Autodesk Inventor part; units mm, degrees
ref_plane "YZ Plane" through (0, 0, 0) normal (1, 0, 0) x (0, 1, 0)
ref_plane "XZ Plane" through (0, 0, 0) normal (0, 1, 0) x (-1, 0, 0)
ref_plane "XY Plane" through (0, 0, 0) normal (0, 0, 1) x (1, 0, 0)
sketch "Sketch_1" plane through (0, 0, 0) normal (0, 0, 1) x (1, 0, 0)
  line L0 (6, 0) -> (-0.8, 0)
  line L1 (-0.8, 0) -> (-0.8, 2.7673)
  line L2 (-0.8, 2.7673) -> (-0.5333, 3.5)
  line L3 (-0.5333, 3.5) -> (0, 3.5)
  line L4 (0, 3.5) -> (0, 1.9)
  arc A0 (0, 1.9) -> (0.4, 1.5) centre (0.4, 1.9) ccw
  line L5 (0.4, 1.5) -> (6, 1.5)
  line L6 (6, 1.5) -> (6, 0)
  line L7 (6, 0) -> (-0.8, 0)
revolve "Revolution1" add sketch "Sketch_1" angle 360 about axis through (6, 0, 0) along (1, 0, 0)
thread "Thread1"
sketch "Sketch_5" plane through (-0.05, 0, 0) normal (1, 0, 0) x (0, 0, -1)
  arc A0 (-0.6801, -0.1159) -> (-0.4404, -0.531) centre (-0.5499, -0.3175) ccw
  arc A1 (-0.341, -0.5357) -> (-0.4404, -0.531) centre (-0.3947, -0.62) ccw
  arc A2 (-0.341, -0.5357) -> (-0.2934, -0.5632) centre (0, 0) ccw
  arc A3 (-0.2397, -0.6469) -> (-0.2934, -0.5632) centre (-0.3396, -0.6519) ccw
  arc A4 (-0.2397, -0.6469) -> (0.2397, -0.6469) centre (0, -0.635) ccw
  arc A5 (0.2934, -0.5632) -> (0.2397, -0.6469) centre (0.3396, -0.6519) ccw
  arc A6 (0.2934, -0.5632) -> (0.341, -0.5357) centre (0, 0) ccw
  arc A7 (0.4404, -0.531) -> (0.341, -0.5357) centre (0.3947, -0.62) ccw
  arc A8 (0.4404, -0.531) -> (0.6801, -0.1159) centre (0.5499, -0.3175) ccw
  arc A9 (0.6344, -0.0275) -> (0.6801, -0.1159) centre (0.7343, -0.0318) ccw
  arc A10 (0.6344, -0.0275) -> (0.6344, 0.0275) centre (0, 0) ccw
  arc A11 (0.6801, 0.1159) -> (0.6344, 0.0275) centre (0.7343, 0.0318) ccw
  arc A12 (0.6801, 0.1159) -> (0.4404, 0.531) centre (0.5499, 0.3175) ccw
  arc A13 (0.341, 0.5357) -> (0.4404, 0.531) centre (0.3947, 0.62) ccw
  arc A14 (0.341, 0.5357) -> (0.2934, 0.5632) centre (0, 0) ccw
  arc A15 (0.2397, 0.6469) -> (0.2934, 0.5632) centre (0.3396, 0.6519) ccw
  arc A16 (0.2397, 0.6469) -> (-0.2397, 0.6469) centre (0, 0.635) ccw
  arc A17 (-0.2934, 0.5632) -> (-0.2397, 0.6469) centre (-0.3396, 0.6519) ccw
  arc A18 (-0.2934, 0.5632) -> (-0.341, 0.5357) centre (0, 0) ccw
  arc A19 (-0.4404, 0.531) -> (-0.341, 0.5357) centre (-0.3947, 0.62) ccw
  arc A20 (-0.4404, 0.531) -> (-0.6801, 0.1159) centre (-0.5499, 0.3175) ccw
  arc A21 (-0.6344, 0.0275) -> (-0.6801, 0.1159) centre (-0.7343, 0.0318) ccw
  arc A22 (-0.6344, 0.0275) -> (-0.6344, -0.0275) centre (0, 0) ccw
  arc A23 (-0.6801, -0.1159) -> (-0.6344, -0.0275) centre (-0.7343, -0.0318) ccw
extrude "Extrusion1" cut sketch "Sketch_5" against normal blind 0.75
sketch "Sketch_2" plane through (0, 0, 0) normal (0, 0, 1) x (1, 0, 0)
  line L0 (0.4552, 0) -> (0, 0)
  line L1 (-0.05, 0) -> (-0.05, 0.875)
  line L2 (-0.05, 0.875) -> (0.4552, 0)
  line L3 (0.4552, 0) -> (-0.05, 0)
revolve "Revolution2" cut sketch "Sketch_2" angle 360 about axis through (0.4552, 0, 0) along (1, 0, 0)
properties part number "超極低頭ネジL6" material "ステンレス鋼"
Work out the finished part from the listing and answer in its coordinate system (mm). A direction names the side the tool comes from. Give positions to 0.01 mm unless a question says otherwise; leave off trailing zeros. Loops run counter-clockwise (first coordinate to the right, second up) from the corner with the lowest first, then second, coordinate; pieces in that order, holes last. Notation, with made-up numbers: (-32.75, 58) - (19.25, 58) arc R25 cw to (19.25, 74) - close; hole circle Ø1 at (32, -28.75). An arc over 180 degrees is marked (long way). Answer in a Markdown table with one row per item. Add a question column.
Q1. The part is cut by section A-A (x = 4). Determine the outline of the cut face in (y, z).
Q2. A tool of negligible diameter and unlimited length cuts with its end or side. For faces 1 (the flat face through (6, 0, 0)), 2 (the flat face through (0, 2, -2)), from which of +Z, -Z, +X, -X, +Y, -Y can it reach the whole face along a straight path? Write none if from no direction.
Q3. The part is cut by section B-B (x = 0.25). Determine the outline of the cut face in (y, z), and give its area (3 significant figures).
Q4. Determine the mould class of faces 3 (the cylindrical face through (3.24, -1.5, 0.07)), 4 (the flat face through (-0.8, 0, 1)), 5 (the conical face through (0.367, -0.033, 0.148)) for opening direction Y: released by +Y, released by -Y, zero draft, split by the parting line, or undercut.
Q5. Each of these flat-tipped pins is pushed along its axis until it touches: P1, Ø3, axis at x = 3, y = 0.5, coming from the +Z side; P2, Ø3, axis at x = 2, z = -0.5, coming from the +Y side; P3, Ø2, axis at y = 1.5, z = 1, coming from the +X side; P4, Ø1, axis at x = 3, y = -1.5, coming from the -Z side. Where does it stop, or does it pass through?
Q6. Consider line 1 along X through (y, z) = (0.25, -2.5); line 2 along Z through (x, y) = (1.25, 0); line 3 along Y through (x, z) = (4.75, -0.5). Determine where each line is inside the solid, lowest interval first.
Solution:
| question | item | result |
|---|---|---|
| 1 | outline | circle Ø3 at (0, 0) |
| 2 | face 1 | +Z, -Z, +X, +Y, -Y |
| 2 | face 2 | +X |
| 3 | outline | circle Ø3.06 at (0, 0); hole circle Ø0.71 at (0, 0) |
| 3 | area | 6.95 mm² |
| 4 | face 3 | split by the parting line |
| 4 | face 4 | zero draft |
| 4 | face 5 | undercut |
| 5 | P1 | stops at z = 1.5 |
| 5 | P2 | stops at y = 1.5 |
| 5 | P3 | stops at x = 6 |
| 5 | P4 | stops at z = -1.12 |
| 6 | line 1 | x = -0.8 to 0 |
| 6 | line 2 | z = -1.5 to 1.5 |
| 6 | line 3 | y = -1.41 to 1.41 |
